Build history of the part. All positions in model axes, mm. A direction names the side the tool comes from. Give positions to 0.01 mm unless a question says otherwise; leave off trailing zeros. Loops run counter-clockwise (first coordinate to the right, second up) from the corner with the lowest first, then second, coordinate; pieces in that order, holes last. Notation, with made-up numbers: (61, -2.75) -> (115, -2.75) arc R27 cw to (115, 19.25) -> close; hole circle Ø11 at (-19.5, 64.25). An arc over 180 degrees is marked (long way). One line per question, with ' | ' between items. Start each with the question number.
(1) Slice it at B-B, the plane x = -22. Write the cut outline in (y, z) (3 decimals).
(2) Slice it at C-C, the plane x = 32.12. Write the cut outline in (y, z) (3 decimals).
(3) Slice it at D-D, the plane y = -15.5. Write the cut outline in (x, z) (1 decimal).
(4) Drill centre lines: L1, parallel to X at y = -3.1, z = -1.98 (3 decimals); L2, parallel to Z at x = -22, y = -8.15; L3, parallel to X at y = -47, z = -5.1. Where is each one in solid material? Low to high. Write a range as from..to.
(5) 3-axis set-ups, long thin cutter, end or side, ignore diameter. For faces 1 (the face through (-11.55, -42.26, -7.57)), 2 (the face through (22, -10, -1)), 3 (the face through (-4.25, -17.6, -0.57)), 4 (the face through (20.78, -1.22, -5.59)), 5 (the face through (18, -6, -11)): which of +Z, -Z, +X, -X, +Y, -Y reach the whole face in a straight line?
(6) Mould opens along X. For faces 6 (the face through (-38.12, -30, -4)), 7 (the face through (2, -30, -18.01)), 8 (the face through (22.067, -34.65, -7.054)) say: pulls with the +X half, pulls with the -X half, needs draft (parallel to the pull), parting line crosses it, or undercut.
(7) Slice it at A-A, the plane y = -26. Write the cut outline in (x, z) (1 decimal).
(8) Flat gauge pins, fed straight in: pin 1 Ø8 at (x, z) = (32.12, -1.98) entering from +Y; pin 2 Ø4.5 at (x, z) = (-22, -4.005) entering from -Y; pin 3 Ø4.5 at (x, y) = (25, -2) entering from +Z; pin 4 Ø3.5 at (x, y) = (0.5, -43.5) entering from +Z. Where does each tip first touch, or does it go through?
```python
from build123d import *

# Parameters (mm, degrees)
SKETCH1_R           = 2
SKETCH1_R_2         = 3.125
SKETCH1_R_3         = 1.7
BOSS_EXTRUDE1_DEPTH = 10
FILLET2_R           = 3
FILLET1_R           = 2
SKETCH1_4_R         = 3.125
CUT_EXTRUDE3_DEPTH  = 5.07
SKETCH1_7_R         = 1.7
CUT_EXTRUDE6_DEPTH  = 10
CUT_EXTRUDE5_DEPTH  = 3
SKETCH1_5_R         = 2
CUT_EXTRUDE4_DEPTH  = 2.48
SKETCH4_R           = 1.5
CUT_EXTRUDE7_DEPTH  = 10
SKETCH5_R           = 2.725
CUT_EXTRUDE8_DEPTH  = 2.8
BOSS_EXTRUDE2_DEPTH = 10
BOSS_EXTRUDE3_DEPTH = 50
FILLET13_R          = 5
CUT_EXTRUDE14_DEPTH = 15
SKETCH10_W          = 8
SKETCH10_H          = 6
CUT_EXTRUDE12_DEPTH = 40
FILLET12_R          = 2
FILLET14_R          = 2
CUT_EXTRUDE17_DEPTH = 20
SKETCH19_R          = 1.5
CUT_EXTRUDE18_DEPTH = 4
CUT_EXTRUDE19_START = 35
SKETCH20_R          = 3
CUT_EXTRUDE19_DEPTH = 109.331401869


with BuildPart() as part:
    # Sketch1 → Boss-Extrude1 (new body)
    with BuildSketch(Plane(origin=(0, 0, 0), x_dir=(1, 0, 0), z_dir=(0, 1, 0))):
        with BuildLine():
            ThreePointArc((-11.409245094, 8.977987014), (-9.849239736, 9.28), (-8.289234378, 8.977987014))
            ThreePointArc((-8.289234378, 8.977987014), (-5.835653376, 8.254222737), (-3.289234378, 8.01))
            Line((-3.289234378, 8.01), (38.12, 8.01))
            Line((38.12, 8.01), (38.12, -3.81))
            Line((38.12, -3.81), (28.478275237, -3.81))
            Line((28.478275237, -3.81), (26.178275237, 0))
            Line((26.178275237, 0), (-26.178275237, 0))
            Line((-26.178275237, 0), (-28.478275237, -3.81))
            Line((-28.478275237, -3.81), (-38.12, -3.81))
            Line((-38.12, -3.81), (-38.12, 8.01))
            Line((-38.12, 8.01), (-16.409245094, 8.01))
            ThreePointArc((-16.409245094, 8.01), (-13.862826096, 8.254222737), (-11.409245094, 8.977987014))
        make_face()
        with Locations((22, 4.005)):
            Circle(SKETCH1_R, mode=Mode.SUBTRACT)
        with Locations((-22, 4.005)):
            Circle(SKETCH1_R, mode=Mode.SUBTRACT)
        with Locations((-32.12, 1.98)):
            Circle(SKETCH1_R_2, mode=Mode.SUBTRACT)
        with Locations((32.12, 1.98)):
            Circle(SKETCH1_R_2, mode=Mode.SUBTRACT)
        with Locations((-9.849239736, 5.1)):
            Circle(SKETCH1_R_3, mode=Mode.SUBTRACT)
        with BuildLine():
            ThreePointArc((11.912105026, 2.53), (14.127105026, 4.745), (11.912105026, 6.96))
            Line((11.912105026, 6.96), (5.992105026, 6.96))
            ThreePointArc((5.992105026, 6.96), (3.777105026, 4.745), (5.992105026, 2.53))
            Line((5.992105026, 2.53), (11.912105026, 2.53))
        make_face(mode=Mode.SUBTRACT)
        with Locations((-22, 4.005)):
            Circle(SKETCH1_R)
        with Locations((-9.849239736, 5.1)):
            Circle(SKETCH1_R_3)
        with Locations((-32.12, 1.98)):
            Circle(SKETCH1_R_2)
        with BuildLine():
            Line((5.992105026, 2.53), (11.912105026, 2.53))
            ThreePointArc((11.912105026, 2.53), (14.127105026, 4.745), (11.912105026, 6.96))
            Line((11.912105026, 6.96), (5.992105026, 6.96))
            ThreePointArc((5.992105026, 6.96), (3.777105026, 4.745), (5.992105026, 2.53))
        make_face()
        with Locations((22, 4.005)):
            Circle(SKETCH1_R)
        with Locations((32.12, 1.98)):
            Circle(SKETCH1_R_2)
    extrude(amount=-BOSS_EXTRUDE1_DEPTH)

    # Fillet2
    fillet2_edges = [part.edges().sort_by_distance(p)[0] for p in [
        (28.478275237, -5, 3.81),
        (-28.478275237, -5, 3.81),
    ]]
    fillet(fillet2_edges, radius=FILLET2_R)

    # Fillet1
    fillet1_edges = [part.edges().sort_by_distance(p)[0] for p in [
        (26.178275237, -5, 0),
        (-26.178275237, -5, 0),
    ]]
    fillet(fillet1_edges, radius=FILLET1_R)

    # Sketch1_4 → Cut-Extrude3 (cut)
    with BuildSketch(Plane(origin=(0, 0, 0), x_dir=(1, 0, 0), z_dir=(0, 1, 0))):
        with Locations(Location((32.12, 1.98, 0), (0, 0, 270))):
            Circle(SKETCH1_4_R)
        with Locations(Location((-32.12, 1.98, 0), (0, 0, 270))):
            Circle(SKETCH1_4_R)
    extrude(amount=-CUT_EXTRUDE3_DEPTH, mode=Mode.SUBTRACT)

    # Sketch1_7 → Cut-Extrude6 (cut)
    with BuildSketch(Plane(origin=(0, 0, 0), x_dir=(1, 0, 0), z_dir=(0, 1, 0))):
        with Locations(Location((-9.849239736, 5.1, 0), (0, 0, 270))):
            Circle(SKETCH1_7_R)
    extrude(amount=-CUT_EXTRUDE6_DEPTH, mode=Mode.SUBTRACT)

    # Sketch1_6 → Cut-Extrude5 (cut)
    with BuildSketch(Plane(origin=(0, 0, 0), x_dir=(1, 0, 0), z_dir=(0, 1, 0))):
        with BuildLine():
            Line((5.992105026, 2.53), (11.912105026, 2.53))
            ThreePointArc((11.912105026, 2.53), (14.127105026, 4.745), (11.912105026, 6.96))
            Line((11.912105026, 6.96), (5.992105026, 6.96))
            ThreePointArc((5.992105026, 6.96), (3.777105026, 4.745), (5.992105026, 2.53))
        make_face()
    extrude(amount=-CUT_EXTRUDE5_DEPTH, mode=Mode.SUBTRACT)

    # Sketch1_5 → Cut-Extrude4 (cut)
    with BuildSketch(Plane(origin=(0, 0, 0), x_dir=(1, 0, 0), z_dir=(0, 1, 0))):
        with Locations(Location((-22, 4.005, 0), (0, 0, 270))):
            Circle(SKETCH1_5_R)
        with Locations(Location((22, 4.005, 0), (0, 0, 270))):
            Circle(SKETCH1_5_R)
    extrude(amount=-CUT_EXTRUDE4_DEPTH, mode=Mode.SUBTRACT)

    # Sketch4 → Cut-Extrude7 (cut)
    with BuildSketch(Plane(origin=(0, 0, 0), x_dir=(1, 0, 0), z_dir=(0, 1, 0))):
        with Locations(Location((-22, 4.005, 0), (0, 0, 270))):
            Circle(SKETCH4_R)
        with Locations(Location((22, 4.005, 0), (0, 0, 270))):
            Circle(SKETCH4_R)
    extrude(amount=-CUT_EXTRUDE7_DEPTH, mode=Mode.SUBTRACT)

    # Sketch5 → Cut-Extrude8 (cut)
    with BuildSketch(Plane.XZ.offset(10)):
        with Locations(Location((22, -4.005, 0), (0, 0, 270))):
            Circle(SKETCH5_R)
        with Locations(Location((-22, -4.005, 0), (0, 0, 90))):
            Circle(SKETCH5_R)
    extrude(amount=-CUT_EXTRUDE8_DEPTH, mode=Mode.SUBTRACT)

    # Sketch6 → Boss-Extrude2 (add)
    with BuildSketch(Plane(origin=(0, 0, 0), x_dir=(1, 0, 0), z_dir=(0, 1, 0))):
        with BuildLine():
            Line((-38.12, 8.01), (-38.12, 18.01))
            Line((-38.12, 18.01), (38.12, 18.01))
            Line((38.12, 18.01), (38.12, 8.01))
            Line((38.12, 8.01), (-3.289234378, 8.01))
            ThreePointArc((-3.289234378, 8.01), (-5.835653376, 8.254222737), (-8.289234378, 8.977987014))
            ThreePointArc((-8.289234378, 8.977987014), (-9.849239736, 9.28), (-11.409245094, 8.977987014))
            ThreePointArc((-11.409245094, 8.977987014), (-13.862826096, 8.254222737), (-16.409245094, 8.01))
            Line((-16.409245094, 8.01), (-38.12, 8.01))
        make_face()
    extrude(amount=-BOSS_EXTRUDE2_DEPTH)

    # Sketch8 → Boss-Extrude3 (add)
    with BuildSketch(Plane.XZ.offset(10)):
        with BuildLine():
            Line((18.950546011, 0), (-18.950546011, 0))
            Line((-18.950546011, 0), (-18.950546011, -4.005))
            ThreePointArc((-18.950546011, -4.005), (-22, -7.054453989), (-25.049453989, -4.005))
            Line((-25.049453989, -4.005), (-25.049453989, 0))
            ThreePointArc((-25.049453989, 0), (-26.032503369, 0.25827272), (-26.761657912, 0.966386084))
            Line((-26.761657912, 0.966386084), (-27.603201224, 2.360420875))
            ThreePointArc((-27.603201224, 2.360420875), (-28.696933037, 3.422590919), (-30.171507108, 3.81))
            Line((-30.171507108, 3.81), (-38.12, 3.81))
            Line((-38.12, 3.81), (-38.12, -18.01))
            Line((-38.12, -18.01), (38.12, -18.01))
            Line((38.12, -18.01), (38.12, 3.81))
            Line((38.12, 3.81), (30.171507108, 3.81))
            ThreePointArc((30.171507108, 3.81), (28.696933037, 3.422590919), (27.603201224, 2.360420875))
            Line((27.603201224, 2.360420875), (26.761657912, 0.966386084))
            ThreePointArc((26.761657912, 0.966386084), (26.032503369, 0.25827272), (25.049453989, 0))
            Line((25.049453989, 0), (25.049453989, -4.005))
            ThreePointArc((25.049453989, -4.005), (22, -7.054453989), (18.950546011, -4.005))
            Line((18.950546011, -4.005), (18.950546011, 0))
        make_face()
    extrude(amount=BOSS_EXTRUDE3_DEPTH)

    # Fillet13
    fillet13_edges = [part.edges().sort_by_distance(p)[0] for p in [
        (-38.12, -30, -18.01),
    ]]
    fillet(fillet13_edges, radius=FILLET13_R)

    # Sketch8_3 → Cut-Extrude14 (cut)
    with BuildSketch(Plane.XZ.offset(10)):
        with BuildLine():
            Line((-4.849239736, 0), (-4.849239736, -5.1))
            ThreePointArc((-4.849239736, -5.1), (-9.849239736, -10.1), (-14.849239736, -5.1))
            Line((-14.849239736, -5.1), (-14.849239736, 0))
            Line((-14.849239736, 0), (-4.849239736, 0))
        make_face()
    extrude(amount=CUT_EXTRUDE14_DEPTH, mode=Mode.SUBTRACT)

    # Sketch10 → Cut-Extrude12 (cut)
    with BuildSketch(Plane(origin=(38.12, 0, 0), x_dir=(0, 0, -1), z_dir=(1, 0, 0))):
        with Locations((12.01, -3)):
            Rectangle(SKETCH10_W, SKETCH10_H)
    extrude(amount=-CUT_EXTRUDE12_DEPTH, mode=Mode.SUBTRACT)

    # Fillet12
    fillet12_edges = [part.edges().sort_by_distance(p)[0] for p in [
        (-4.849239736, -17.5, 0),
        (-14.849239736, -17.5, 0),
    ]]
    fillet(fillet12_edges, radius=FILLET12_R)

    # Fillet14
    fillet14_edges = [part.edges().sort_by_distance(p)[0] for p in [
        (-1.88, -3, -16.01),
        (18.12, -6, -16.01),
        (-1.88, -3, -8.01),
    ]]
    fillet(fillet14_edges, radius=FILLET14_R)

    # Sketch18 → Cut-Extrude17 (cut)
    with BuildSketch(Plane.XZ.offset(60)):
        Polygon((-10, 0), (-10, -3), (-12.5, -3), (-12.5, -6), (12.5, -6), (12.5, -3), (10, -3), (10, 0), align=None)
    extrude(amount=-CUT_EXTRUDE17_DEPTH, mode=Mode.SUBTRACT)

    # Sketch19 → Cut-Extrude18 (cut)
    with BuildSketch(Plane.XY.offset(-6)):
        with Locations((0, -44)):
            Circle(SKETCH19_R)
    extrude(amount=-CUT_EXTRUDE18_DEPTH, mode=Mode.SUBTRACT)

    # Sketch20 → Cut-Extrude19 (cut, through all)
    with BuildSketch(Plane(origin=(0, -60, 0), x_dir=(1, 0, 0), z_dir=(0, 1, 0)).offset(CUT_EXTRUDE19_START)):
        with Locations(Location((-9.849239736, 5.1, 0), (0, 0, 267.119477763))):
            Circle(SKETCH20_R)
    extrude(amount=-CUT_EXTRUDE19_DEPTH, mode=Mode.SUBTRACT)


solid = part.part
```
Final values:
1) outline: (-60, -18.01) -> (0, -18.01) -> (0, -6.005) -> (-2.48, -6.005) -> (-2.48, -5.505) -> (-7.2, -5.505) -> (-7.2, -6.73) -> (-10, -6.73) -> (-10, -7.054) -> (-60, -7.054) -> close; (-10, -1.28) -> (-7.2, -1.28) -> (-7.2, -2.505) -> (-2.48, -2.505) -> (-2.48, -2.005) -> (0, -2.005) -> (0, 0) -> (-10, 0) -> close
2) outline: (-60, -18.01) -> (0, -18.01) -> (0, -16.01) -> (-4, -16.01) arc R2 cw to (-6, -14.01) -> (-6, -8.01) -> (0, -8.01) -> (0, -5.105) -> (-5.07, -5.105) -> (-5.07, 1.145) -> (0, 1.145) -> (0, 3.81) -> (-60, 3.81) -> close
3) outline: (-38.1, -13) arc R5 ccw to (-33.1, -18) -> (38.1, -18) -> (38.1, 3.8) -> (30.2, 3.8) arc R3 ccw to (27.6, 2.4) -> (26.8, 1) arc R2 cw to (25, 0) -> (25, -4) arc R3 cw to (19, -4) -> (19, 0) -> (-2.8, 0) arc R2 ccw to (-4.8, -2) -> (-4.8, -5.1) arc R5 cw to (-14.8, -5.1) -> (-14.8, -2) arc R2 ccw to (-16.8, 0) -> (-19, 0) -> (-19, -4) arc R3 cw to (-25, -4) -> (-25, 0) arc R2 cw to (-26.8, 1) -> (-27.6, 2.4) arc R3 ccw to (-30.2, 3.8) -> (-38.1, 3.8) -> close
4) L1: -38.12..-35.245, -28.995..28.995, 35.245..38.12 | L2: -18.01..-6.73, -1.28..0 | L3: -38.12..-24.85, -19.15..-12.85, 12.5..19.15, 24.85..38.12
5) face 1: -Y | face 2: +Z, -Y | face 3: +Z | face 4: +Y | face 5: +X, +Y
6) face 6: pulls with the -X half | face 7: needs draft | face 8: undercut
7) outline: (-38.1, -13) arc R5 ccw to (-33.1, -18) -> (38.1, -18) -> (38.1, 3.8) -> (30.2, 3.8) arc R3 ccw to (27.6, 2.4) -> (26.8, 1) arc R2 cw to (25, 0) -> (25, -4) arc R3 cw to (19, -4) -> (19, 0) -> (-19, 0) -> (-19, -4) arc R3 cw to (-25, -4) -> (-25, 0) arc R2 cw to (-26.8, 1) -> (-27.6, 2.4) arc R3 ccw to (-30.2, 3.8) -> (-38.1, 3.8) -> close; hole circle Ø6 at (-9.8, -5.1)
8) pin 1: y = 0 | pin 2: y = -7.2 | pin 3: z = 1.78 | pin 4: z = -6
